Source: CAD feature listing. Evaluate the final solid. Frame: model axes, mm. A direction names the side the tool comes from. Coordinates: 2 decimals unless noted, no trailing zeros. Write each loop counter-clockwise with the first axis right and the second up, starting at its lowest first coordinate (ties: lowest second). Pieces come first, ordered by that corner, then holes. Notation, with made-up numbers: (-13, 77.5) -> (-1, 77.5) arc R25 cw to (-1, 96.5) -> close; hole circle Ø11 at (-26.5, 66). An arc over 180 degrees is marked (long way). One line per item, written item: value. Start each with the question number.
1. Line query: line 1 (X direction, y = 0, z = 1.25); line 2 (X direction, y = -25, z = -1.75); line 3 (X direction, y = -17.5, z = -3.5). Output: solid intervals per line, ascending.
2. Section query B-B, the plane x = 0. Output: boundary loops of the cut face in (y, z).
3. Section query C-C, the plane y = -15. Output: boundary loops of the cut face in (x, z).
4. Section query A-A, the plane y = 0. Output: boundary loops of the cut face in (x, z), and give its area (3 significant figures).
5. Access query for faces 1 (the flat face through (8.357, -17.915, -3.658)), 2 (the flat face through (-7, -18, 1.25)), 3 (the flat face through (2, -14.294, 0)). Directions: +Z, -Z, +X, -X, +Y, -Y. A direction counts if a zero-diameter tool reaches every point of the face in a straight line with its end or side. Return the directions, or none.
6. Mould query, pull axis Y, two halves, no side actions, for faces 4 (the flat face through (-7, -18, -1.25)), 5 (the flat face through (0, -11, -6)), 6 (the flat face through (11.177, -15.492, 0.084)). Classes: released by +Y, released by -Y, zero draft, split by the parting line, or undercut.
7. Section query D-D, the plane z = 0. Output: boundary loops of the cut face in (x, y), and give its area (3 significant figures).
8. First-contact query: P1, Ø1.2, axis at x = -7.5, y = -17.5, coming from the -Z side; P2, Ø1.4, axis at x = 1.5, z = -2.5, coming from the +Y side (3 decimals); P3, Ø10, axis at x = 1.5, y = -18.5, coming from the -Z side. Flat tips, straight axial feed; report the tip coordinate or a pass-through.
from build123d import *

# Parameters (mm, degrees)
BOSS_EXTRUDE1_DEPTH      = 6
CUT_EXTRUDE1_DEPTH       = 4.75
BOSS_EXTRUDE2_REACH      = 42.608
BOSS_EXTRUDE2_END_RADIUS = 12.5
SKETCH5_R                = 5.5
FILLET1_R                = 0.5
CUT_EXTRUDE2_DEPTH       = 5
CUT_EXTRUDE2_DEPTH_BACK  = 3
SKETCH6_R                = 3
SKETCH7_R                = 1.7
CUT_EXTRUDE3_DEPTH       = 28.342769961


with BuildPart() as part:
    # Sketch1 → Boss-Extrude1 (new, symmetric)
    with BuildSketch(Plane.XY):
        with BuildLine():
            Line((-9.5, -29), (9.5, -29))
            Line((9.5, -29), (12.900989015, -1.60140015))
            ThreePointArc((12.900989015, -1.60140015), (12.444176754, 3.760646876), (9.854901959, 8.47826087))
            ThreePointArc((9.854901959, 8.47826087), (7.739537018, 8.637104072), (7.580693815, 6.52173913))
            ThreePointArc((7.580693815, 6.52173913), (0, -10), (-7.580693815, 6.52173913))
            ThreePointArc((-7.580693815, 6.52173913), (-7.739537018, 8.637104072), (-9.854901959, 8.47826087))
            ThreePointArc((-9.854901959, 8.47826087), (-12.444176754, 3.760646876), (-12.900989015, -1.60140015))
            Line((-12.900989015, -1.60140015), (-9.5, -29))
        make_face()
    extrude(amount=BOSS_EXTRUDE1_DEPTH, both=True)

    # Sketch2 → Cut-Extrude1 (cut)
    with BuildSketch(Plane.XY.offset(6)):
        with BuildLine():
            Line((-9.5845508, -8.024112783), (-7.29113837, -26.5))
            Line((-7.29113837, -26.5), (7.29113837, -26.5))
            Line((7.29113837, -26.5), (9.5845508, -8.024112783))
            ThreePointArc((9.5845508, -8.024112783), (0, -12.5), (-9.5845508, -8.024112783))
        make_face()
    cut_extrude1 = extrude(amount=-CUT_EXTRUDE1_DEPTH, mode=Mode.SUBTRACT)

    # Mirror1: Cut-Extrude1 across plane
    add(cut_extrude1.mirror(Plane.XY), mode=Mode.SUBTRACT)

    # Boss-Extrude2: up to this cylinder (the profile starts outside it)
    boss_extrude2_end = Plane(origin=(0, 0, 0), z_dir=(0, 0, 1)) * Cylinder(BOSS_EXTRUDE2_END_RADIUS, 111.216, mode=Mode.PRIVATE)
    # Sketch5 → Boss-Extrude2 (add, up to the surface)
    with BuildSketch(Plane.XZ.offset(29), mode=Mode.PRIVATE) as boss_extrude2_sk1:
        Circle(SKETCH5_R)
    boss_extrude2_tool1 = extrude(boss_extrude2_sk1.sketch, amount=-BOSS_EXTRUDE2_REACH, mode=Mode.PRIVATE) - boss_extrude2_end
    add(boss_extrude2_tool1.solids().sort_by_distance((0, -29, 0))[0])

    # Fillet1
    fillet1_edges = [part.edges().sort_by_distance(p)[0] for p in [
        (-9.5845508, -8.024112783, 3.625),
        (9.5845508, -8.024112783, 3.625),
        (7.29113837, -26.5, 3.625),
        (-7.29113837, -26.5, 3.625),
        (9.5845508, -8.024112783, -3.625),
        (-9.5845508, -8.024112783, -3.625),
        (-7.29113837, -26.5, -3.625),
        (7.29113837, -26.5, -3.625),
    ]]
    fillet(fillet1_edges, radius=FILLET1_R)

    # Sketch6 → Cut-Extrude2 (cut, two sides: drawn at the far end of the back side and taken through both)
    with BuildSketch(Plane(origin=(0, -11.294356998, 0), x_dir=(1, 0, 0), z_dir=(0, 1, 0)).offset(-CUT_EXTRUDE2_DEPTH_BACK)):
        with Locations(Location((0, 0, 0), (0, 0, 90))):
            Circle(SKETCH6_R)
    extrude(amount=CUT_EXTRUDE2_DEPTH + CUT_EXTRUDE2_DEPTH_BACK, mode=Mode.SUBTRACT)

    # Sketch7 → Cut-Extrude3 (cut, through all)
    with BuildSketch(Plane(origin=(0, -14.294356998, 0), x_dir=(1, 0, 0), z_dir=(0, 1, 0))):
        with Locations(Location((0, 0, 0), (0, 0, 270))):
            Circle(SKETCH7_R)
    extrude(amount=-CUT_EXTRUDE3_DEPTH, mode=Mode.SUBTRACT)


solid = part.part
Computed values:
1. line 1: x = -13 to -10, 10 to 13
1. line 2: x = -10 to -7.48, -5.21 to 5.21, 7.48 to 10
1. line 3: x = -10.93 to -8.41, -4.24 to 4.24, 8.41 to 10.93
2. outline: (-29, -6) -> (-26.5, -6) -> (-26.5, -5.5) -> (-12.5, -5.5) -> (-12.5, -6) -> (-10, -6) -> (-10, -3) -> (-14.29, -3) -> (-14.29, -1.7) -> (-29, -1.7) -> close; (-29, 1.7) -> (-14.29, 1.7) -> (-14.29, 3) -> (-10, 3) -> (-10, 6) -> (-12.5, 6) -> (-12.5, 5.5) -> (-26.5, 5.5) -> (-26.5, 6) -> (-29, 6) -> close
3. outline: (-11.24, -6) -> (-8.72, -6) -> (-8.72, -1.25) -> (-5.36, -1.25) arc R5.5 ccw to (5.36, -1.25) -> (8.72, -1.25) -> (8.72, -6) -> (11.24, -6) -> (11.24, 6) -> (8.72, 6) -> (8.72, 1.25) -> (5.36, 1.25) arc R5.5 ccw to (-5.36, 1.25) -> (-8.72, 1.25) -> (-8.72, 6) -> (-11.24, 6) -> close; hole circle Ø3.4 at (0, 0)
4. outline: (-13, -6) -> (-10, -6) -> (-10, 6) -> (-13, 6) -> close; (10, -6) -> (13, -6) -> (13, 6) -> (10, 6) -> close
4. area: 72.0 mm²
5. face 1: -Z
5. face 2: +Z
5. face 3: +Y
6. face 4: undercut
6. face 5: zero draft
6. face 6: released by -Y
7. outline: (-12.9, -1.6) -> (-9.5, -29) -> (-1.7, -29) -> (-1.7, -14.29) -> (-3, -14.29) -> (-3, -9.54) arc R10 cw to (-7.58, 6.52) arc R1.5 ccw to (-9.85, 8.48) arc R13 ccw to start; (1.7, -29) -> (9.5, -29) -> (12.9, -1.6) arc R13 ccw to (9.85, 8.48) arc R1.5 ccw to (7.58, 6.52) arc R10 cw to (3, -9.54) -> (3, -14.29) -> (1.7, -14.29) -> close
7. area: 478 mm²
8. P1: stops at z = -1.25
8. P2: stops at y = -9.755
8. P3: stops at z = -5.5
